Model file for the job. Use its own axes, mm. Face numbers are marked on the shaded views. Round coordinates to 2 decimals unless told otherwise and drop trailing zeros. Loops run counter-clockwise (first coordinate to the right, second up) from the corner with the lowest first, then second, coordinate; pieces in that order, holes last. Notation, with made-up numbers: (59.25, -14.75) -> (68.25, -14.75) arc R15 ccw to (68.25, 14.25) -> close; hole circle Ø10 at (-36, 20). An arc over 180 degrees is marked (long way). Use a Markdown table: item, result. Add a question column.
```python
from build123d import *

# Parameters (mm, degrees)
SKETCH1_R          = 25
BASE_FLANGE1_DEPTH = 40
SKETCH8_R          = 11
CUT_EXTRUDE2_DEPTH = 5
SKETCH9_R          = 7.5
CUT_EXTRUDE3_DEPTH = 50.749371855


# Sheet-metal steps are written as plain solids
with BuildPart() as part:
    # Sketch1 → Base-Flange1 (new body)
    with BuildSketch(Plane(origin=(0, 0, 0), x_dir=(1, 0, 0), z_dir=(0, 1, 0))):
        with Locations(Location((0, 0, 0), (0, 0, 270))):
            Circle(SKETCH1_R)
    extrude(amount=-BASE_FLANGE1_DEPTH)

    # Sketch8 → Cut-Extrude2 (cut)
    with BuildSketch(Plane.XZ.offset(40)):
        with Locations(Location((0, 0, 0), (0, 0, 270))):
            Circle(SKETCH8_R)
    extrude(amount=-CUT_EXTRUDE2_DEPTH, mode=Mode.SUBTRACT)

    # Sketch9 → Cut-Extrude3 (cut, through all)
    with BuildSketch(Plane.XZ.offset(35)):
        with Locations(Location((0, 0, 0), (0, 0, 270))):
            Circle(SKETCH9_R)
    extrude(amount=-CUT_EXTRUDE3_DEPTH, mode=Mode.SUBTRACT)


solid = part.part
```
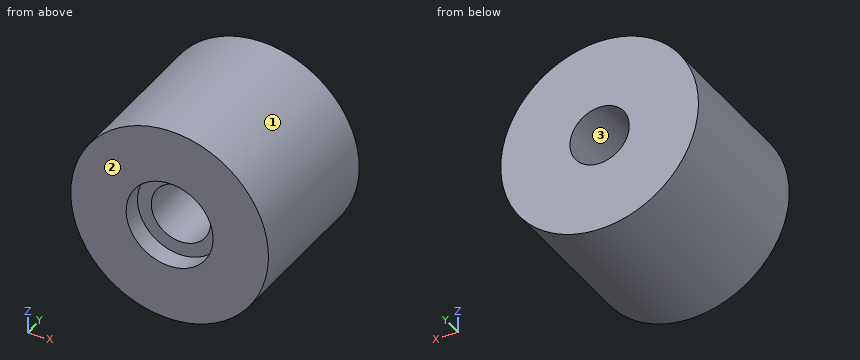
1) Wall check: probe 1 along X at (y, z) = (-28, 0); probe 2 along X at (y, z) = (-38.45, 0); probe 3 along Z at (x, y) = (-1.5, -8.5). Give the ranges that are in metal, low to high. Write a range as from..to.
2) Cut at C-C on y = -11. Write the cut outline in (x, z).
3) Cut at D-D on x = 20. Write the cut outline in (y, z), and give its area (3 significant figures).
4) Cut at B-B on x = 0. Write the cut outline in (y, z).
5) Cut at A-A on z = 0. Write the cut outline in (x, y), and give its area (4 significant figures).
6) Pin check, flat tips, straight feed: pin 1 Ø2 at (x, y) = (-6.5, -28.5) entering from +Z; pin 2 Ø2 at (y, z) = (-31, -3.5) entering from -X; pin 3 Ø5 at (x, y) = (-15, -29.5) entering from +Z. Stop position of each tip, or through.
7) Pull direction X, two halves, no side cores. Call the marked faces 1, 2 and 3: +X half, -X half, draft (parallel to the pull), parting line (faces both ways), or undercut.
Established:
| question | item | result |
|---|---|---|
| 1 | probe 1 | x = -25..-7.5, 7.5..25 |
| 1 | probe 2 | x = -25..-11, 11..25 |
| 1 | probe 3 | z = -24.95..-7.35, 7.35..24.95 |
| 2 | outline | circle Ø50 at (0, 0); hole circle Ø15 at (0, 0) |
| 3 | outline | (-40, -15) -> (0, -15) -> (0, 15) -> (-40, 15) -> close |
| 3 | area | 1,200 mm^2 |
| 4 | outline | (-40, -25) -> (0, -25) -> (0, -7.5) -> (-35, -7.5) -> (-35, -11) -> (-40, -11) -> close; (-40, 11) -> (-35, 11) -> (-35, 7.5) -> (0, 7.5) -> (0, 25) -> (-40, 25) -> close |
| 5 | outline | (-25, -40) -> (-11, -40) -> (-11, -35) -> (-7.5, -35) -> (-7.5, 0) -> (-25, 0) -> close; (7.5, -35) -> (11, -35) -> (11, -40) -> (25, -40) -> (25, 0) -> (7.5, 0) -> close |
| 5 | area | 1,365 mm^2 |
| 6 | pin 1 | stops at z = 24.39 |
| 6 | pin 2 | stops at x = -24.87 |
| 6 | pin 3 | stops at z = 21.65 |
| 7 | face 1 | parting line |
| 7 | face 2 | draft |
| 7 | face 3 | undercut |
